```python
from build123d import *

# Parameters (mm, degrees)
SKETCH1_W           = 296
SKETCH1_H           = 496
SKETCH1_R           = 11
SKETCH1_R_2         = 22
SKETCH1_R_3         = 3
SKETCH1_W_2         = 45.5
SKETCH1_H_2         = 45.5
BOSS_EXTRUDE1_DEPTH = 2


with BuildPart() as part:
    # Sketch1 → Boss-Extrude1 (new body)
    with BuildSketch(Plane.XY):
        Rectangle(SKETCH1_W, SKETCH1_H)
        with Locations((-74, 99.5)):
            Circle(SKETCH1_R, mode=Mode.SUBTRACT)
        with Locations((-74, 198.5)):
            Circle(SKETCH1_R_2, mode=Mode.SUBTRACT)
        with Locations((-138, 238)):
            Circle(SKETCH1_R_3, mode=Mode.SUBTRACT)
        with Locations((138, 238)):
            Circle(SKETCH1_R_3, mode=Mode.SUBTRACT)
        with Locations((-138, -238)):
            Circle(SKETCH1_R_3, mode=Mode.SUBTRACT)
        with Locations((138, -238)):
            Circle(SKETCH1_R_3, mode=Mode.SUBTRACT)
        with Locations((74, 198.5)):
            Rectangle(SKETCH1_W_2, SKETCH1_H_2, mode=Mode.SUBTRACT)
        with Locations((74, 99.5)):
            Rectangle(SKETCH1_W_2, SKETCH1_H_2, mode=Mode.SUBTRACT)
    extrude(amount=BOSS_EXTRUDE1_DEPTH)


solid = part.part
```
Input: part model. Units: mm. Frame: model coordinates. Coordinates: 2 decimals unless noted, no trailing zeros. Loops run counter-clockwise (first coordinate to the right, second up) from the corner with the lowest first, then second, coordinate; pieces in that order, holes last. Notation, with made-up numbers: M 64.5,41.5 L 82.5,41.5 A20 ccw 82.5,68.5 Z; hole C 28,26.25 d2. An arc over 180 degrees is marked long. Use a Markdown table: item, result. Add a question column.
1) Section A-A, the plane x = -74. Return the cut outline in (y, z), plus the area to 3 significant figures.
2) Section C-C, the plane y = 99.5. Return the cut outline in (x, z).
3) Draft query along Y for faces 1 (the cylindrical face through (-62.17, 217.05, 0.99)), 2 (the flat face through (-2, 3, 2)). Return one class per face: +Y half, -Y half, draft (parallel to the pull), parting line (faces both ways), or undercut.
4) Section B-B, the plane z = 0.85. Give the number of separate pieces and of enclosed holes in the cut face, plus the area to 3 significant figures.
5) Line query: L1, parallel to Y at x = -138, z = 1.1; L2, parallel to X at y = 238, z = 1.55; L3, parallel to Y at x = 71.5, z = 1.4. Output: solid intervals per line, ascending. Write a range as from..to.
Answer below:
| question | item | result |
|---|---|---|
| 1 | outline | M -248,0 L 88.5,0 L 88.5,2 L -248,2 Z; M 110.5,0 L 176.5,0 L 176.5,2 L 110.5,2 Z; M 220.5,0 L 248,0 L 248,2 L 220.5,2 Z |
| 1 | area | 860 mm2 |
| 2 | outline | M -148,0 L -85,0 L -85,2 L -148,2 Z; M -63,0 L 51.25,0 L 51.25,2 L -63,2 Z; M 96.75,0 L 148,0 L 148,2 L 96.75,2 Z |
| 3 | face 1 | undercut |
| 3 | face 2 | draft |
| 4 | separate pieces | 1 |
| 4 | enclosed holes | 8 |
| 4 | area | 141,000 mm2 |
| 5 | L1 | -248..-241, -235..235, 241..248 |
| 5 | L2 | -148..-141, -135..135, 141..148 |
| 5 | L3 | -248..76.75, 122.25..175.75, 221.25..248 |
